For this review, take the finished solid that the model builds, in its own axes (mm). Face numbers are marked on the shaded views. A direction names the side the tool comes from. Coordinates: 2 decimals unless noted, no trailing zeros. Loops run counter-clockwise (first coordinate to the right, second up) from the corner with the lowest first, then second, coordinate; pieces in that order, holes last. Notation, with made-up numbers: (-23.75, -18.5) - (-3.75, -18.5) arc R27 ccw to (-3.75, 17.5) - close; hole circle Ø2 at (7.5, 30.25). An arc over 180 degrees is marked (long way). Answer as a JSON object with one key per item and string values. Group by question number.
Item 1: Tool access review of the marked faces 1, 2, 3 and 4: name each direction out of +Z, -Z, +X, -X, +Y, -Y from which nothing blocks a thin tool from reaching the whole face with its end or side.
Item 2: We need section A-A (x = 11.25). Give the boundary of the cut face in (y, z).
Item 3: We need section B-B (x = 14). Give the boundary of the cut face in (y, z).
Item 4: To check wall thickness, follow line 1 (X direction, y = 2, z = -16); line 2 (X direction, y = 19.9, z = -16); line 3 (Z direction, x = 14, y = 21.9). State the ranges of each line that lie inside material, in increasing order.
Item 5: Mouldability with a two-part tool opening along Z and no side actions: class the marked faces 5, 6 and 7 as released by +Z, released by -Z, zero draft, split by the parting line, or undercut.
Item 6: Clearance check with flat-ended pins moving along their axes: pin 1 (3 mm diameter, centred on x = 14, z = -16, fed in from -Y); pin 2 (6 mm diameter, centred on x = 17, z = -14.5, fed in from +Y); pin 3 (6 mm diameter, centred on x = 16.5, y = 10, fed in from +Z); pin 4 (6 mm diameter, centred on x = 11, z = -15, fed in from +Y). State where each tip first meets the part, or that it passes through.
Item 7: We need section C-C (z = -16). Give the boundary of the cut face in (x, y), then the cut area to 3 significant figures.
Item 8: We need section D-D (y = 9.25). Give the boundary of the cut face in (x, z).
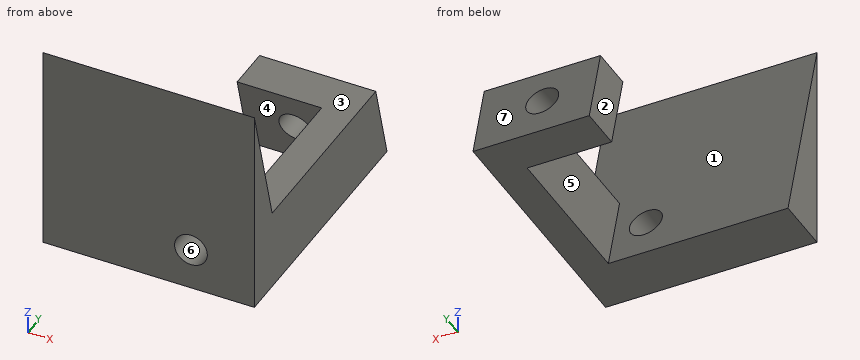
from build123d import *

# Parameters (mm, degrees)
EXTRUDE_3_DEPTH     = 20
EXTRUDE_START       = -3
EXTRUDE_4_DEPTH     = 3
EXTRUDE_7_DEPTH     = 8
SKETCH_13_R         = 1.55
CUT_EXTRUDE_2_DEPTH = 30


# Read off the part's stored shape, not the designer's step: 凸台-拉伸4
with BuildPart() as part:
    # 草图3 → 凸台-拉伸3 (new body)
    with BuildSketch(Plane(origin=(0, 0, 0), x_dir=(0, 0, -1), z_dir=(1, 0, 0))):
        Polygon((0, 0), (20, 0), (20, 5.358983849), align=None)
    extrude(amount=EXTRUDE_3_DEPTH)

    # 凸台-拉伸4 outline → 凸台-拉伸4 (add)
    with BuildSketch(Plane(origin=(20, 0, 0), x_dir=(0, 0, -1), z_dir=(1, 0, 0)).offset(EXTRUDE_START)):
        Polygon((20, 5.358983849), (20, 24.511593186), (12.27259339, 22.441040825), (12.27259339, 3.288431488), align=None)
    extrude(amount=EXTRUDE_4_DEPTH)

    # 草图9 → 凸台-拉伸7 (add)
    with BuildSketch(Plane.ZY.offset(-17)):
        Polygon((-20, 24.511593186), (-12.27259339, 22.441040825), (-12.27259339, 18.299936104), (-20, 20.370488465), align=None)
    extrude(amount=EXTRUDE_7_DEPTH)

    # 草图13 → 切除-拉伸2 (cut)
    with BuildSketch(Plane.XZ):
        with Locations(Location((14, -16, 0), (0, 0, 90))):
            Circle(SKETCH_13_R)
    extrude(amount=-CUT_EXTRUDE_2_DEPTH, mode=Mode.SUBTRACT)


solid = part.part
Check sheet entries:
{
 "1": {"face 1": "+Z, -X", "face 2": "+Z, -Z, -X, +Y", "face 3": "+Z, +X, -X, +Y", "face 4": "-Z, -X"},
 "2": {"outline": "(0, -20) - (5.36, -20) - (0, 0) - close; (18.3, -12.27) - (20.37, -20) - (24.51, -20) - (22.44, -12.27) - close"},
 "3": {"outline": "(0, -20) - (5.36, -20) - (4.7, -17.55) - (0, -17.55) - close; (0, -14.45) - (3.87, -14.45) - (0, 0) - close; (18.3, -12.27) - (18.88, -14.45) - (23.02, -14.45) - (22.44, -12.27) - close; (19.71, -17.55) - (20.37, -20) - (24.51, -20) - (23.86, -17.55) - close"},
 "4": {"line 1": "x = 0 to 12.45, 15.55 to 20", "line 2": "x = 9 to 12.45, 15.55 to 20", "line 3": "z = -20 to -17.55, -14.45 to -12.27"},
 "5": {"face 5": "zero draft", "face 6": "undercut", "face 7": "released by +Z"},
 "6": {"pin 1": "passes through", "pin 2": "stops at y = 23.84", "pin 3": "stops at z = -12.27", "pin 4": "stops at y = 23.98"},
 "7": {"outline": "(0, 0) - (12.45, 0) - (12.45, 4.29) - (0, 4.29) - close; (9, 19.3) - (12.45, 19.3) - (12.45, 23.44) - (9, 23.44) - close; (15.55, 0) - (20, 0) - (20, 23.44) - (15.55, 23.44) - (15.55, 19.3) - (17, 19.3) - (17, 4.29) - (15.55, 4.29) - close", "area": "150 mm2"},
 "8": {"outline": "(17, -20) - (20, -20) - (20, -12.27) - (17, -12.27) - close"}
}
